Source: CAD feature listing. Evaluate the final solid. Frame: model axes, mm. Face numbers are marked on the shaded views. A direction names the side the tool comes from. Give positions to 0.01 mm unless a question says otherwise; leave off trailing zeros. Order: outer loops, then holes, each group sorted by start corner. A loop starts at its lowest first (then second) coordinate and runs counter-clockwise, first axis right, second up. Notation, with made-up numbers: (74, -17.75) -> (99, -17.75) arc R18 ccw to (99, 7.25) -> close; hole circle Ø1 at (85, 14.5). An arc over 180 degrees is marked (long way). Answer in a Markdown table with one row per item.
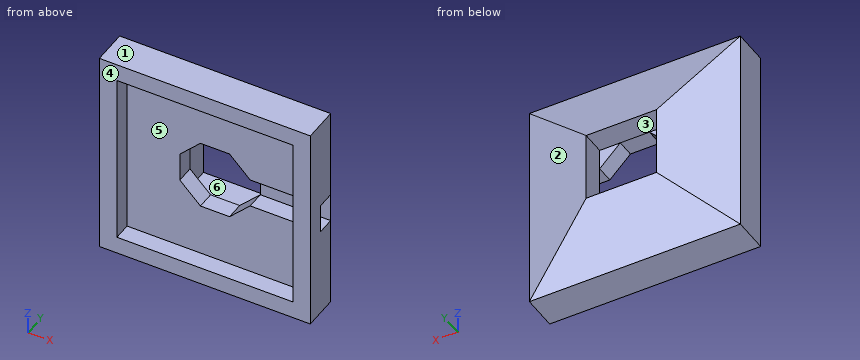
Autodesk Inventor part; units mm, degrees
ref_plane "YZ Plane" through (0, 0, 0) normal (1, 0, 0) x (0, 1, 0)
ref_plane "XZ Plane" through (0, 0, 0) normal (0, 1, 0) x (-1, 0, 0)
ref_plane "XY Plane" through (0, 0, 0) normal (0, 0, 1) x (1, 0, 0)
sketch "Sketch1" plane through (0, 0, 0) normal (0, 1, 0) x (-1, 0, 0)
  line L0 (5, 5) -> (-5, 5)
  line L1 (-5, 5) -> (-5, -5)
  line L2 (-5, -5) -> (5, -5)
  line L3 (5, -5) -> (5, 5)
  line L4 (6, 6) -> (-6, 6)
  line L5 (-6, 6) -> (-6, -6)
  line L6 (-6, -6) -> (6, -6)
  line L7 (6, -6) -> (6, 6)
  point P0 (0, 0)
  dimension "d0" = 10
  dimension "d1" = 10
  dimension "d2" = 5
  dimension "d3" = 5
  dimension "d4" = 12
  dimension "d5" = 12
  dimension "d6" = 1
  dimension "d7" = 1
extrude "Extrusion1" add sketch "Sketch1" along normal blind 2
sketch "Sketch2" plane through (6, 0, 6) normal (1, 0, 0) x (0, 0, -1)
  line L0 (0, 0) -> (0, 2)
  line L1 (12, 0) -> (12, 2)
  line L2 (0, 2) -> (12, 2)
  line L3 (12, 2) -> (12, 1)
  line L4 (12, 1) -> (0, 1)
  line L5 (0, 1) -> (0, 2)
  point P0 (6, 0)
extrude "Extrusion2" add sketch "Sketch2" against normal blind 11.5
sketch "Sketch3" plane through (0, 2, 0) normal (0, 1, 0) x (1, 0, 0)
  line L0 (-2, -2) -> (2, -2)
  line L1 (2, -2) -> (2, 2)
  line L2 (2, 2) -> (-2, 2)
  line L3 (-2, 2) -> (-2, -2)
  circle A0 centre (0, 0) radius 2.8284
  line L4 (0, -2.8284) -> (-2.8284, 0)
  line L5 (-2.8284, 0) -> (0, 2.8284)
  line L6 (2.8284, 0) -> (0, 2.8284)
  line L7 (2.8284, 0) -> (0, -2.8284)
  point P0 (0.8284, -2)
  point P1 (2, -0.8284)
  point P2 (2, 0.8284)
  point P3 (0.8284, 2)
  point P4 (-0.8284, 2)
  point P5 (-2, 0.8284)
  point P6 (-2, -0.8284)
  point P7 (-0.8284, -2)
  dimension "d13" = 4
  dimension "d14" = 4
  dimension "d15" = 2
  dimension "d16" = 2
extrude "Extrusion3" cut sketch "Sketch3" along normal blind 23.25 and the other way blind 11.625 contours L4 L3 L5 L2 L6 L1 L7 L0
sketch "Sketch4" plane through (0, 2, 0) normal (0, 1, 0) x (1, 0, 0)
  line L0 (2, -0.8284) -> (2, 0.8284)
  line L1 (2, -0.8284) -> (2.8765, -0.8284)
  line L2 (2.8765, -0.8284) -> (2.8765, 0.8284)
  line L3 (2.8765, 0.8284) -> (2, 0.8284)
  line L4 (2, 0.8284) -> (2, -0.8284)
  line L5 (2.8765, -0.8284) -> (7.5124, -0.8284)
  line L6 (7.5124, -0.8284) -> (7.5124, 0.8284)
  line L7 (7.5124, 0.8284) -> (2.8765, 0.8284)
  line L8 (2.8765, 0.8284) -> (2.8765, -0.8284)
  point P0 (0, 0)
  point P1 (2.8765, 0.8284)
  point P2 (2, 0.8284)
extrude "Extrusion4" cut sketch "Sketch4" against normal blind 1
sketch "Sketch5" plane through (0, 2, 0) normal (0, 1, 0) x (1, 0, 0)
  line L0 (-6, -6) -> (6, -6)
  line L1 (6, 0.8284) -> (6, 6)
  line L2 (-6, -6) -> (6, -6)
  line L3 (6, -6) -> (6, 6)
  line L4 (6, 6) -> (-6, 6)
  line L5 (-6, 6) -> (-6, -6)
  point P0 (0, 0)
  point P1 (6, -6)
extrude "Extrusion5" add sketch "Sketch5" along normal blind 25
sketch "Sketch6" plane through (6, 0, 6) normal (1, 0, 0) x (0, 0, -1)
  line L0 (5.1716, 1) -> (5.1716, 2)
  line L1 (5.1716, 2) -> (-3.596, 2)
  line L2 (0, 0) -> (0, 27)
  line L3 (4, 2) -> (5.1716, 2)
  line L4 (5.1716, 2) -> (16.1787, 2)
  line L5 (5.1716, 2) -> (6.8284, 2)
  line L6 (6, 2) -> (6, 6)
  line L7 (0, 2) -> (6, 4)
  line L8 (6, 4) -> (12, 2)
  line L9 (12, 0) -> (12, 27)
  line L10 (12, 2) -> (-2.4689, 2)
  line L11 (-2.4689, 2) -> (-2.4689, 28.669)
  line L12 (-2.4689, 28.669) -> (12, 28.669)
  line L13 (12, 28.669) -> (12, 2)
  point P0 (6, 0)
  dimension "d23" = 4
extrude "Extrusion6" cut sketch "Sketch6" against normal blind 23.25 contours L1 L11 L12 L13 L9 L8 L7
sketch "Sketch7" plane through (-6, 0, 6) normal (0, 0, 1) x (1, 0, 0)
  line L0 (6, 0) -> (6, 4)
  line L1 (12, 4) -> (0, 4)
  line L2 (0, 2) -> (12, 2)
  line L3 (12, 2) -> (6, 4)
  line L4 (0, 4) -> (0, 2)
  line L5 (6, 4) -> (0, 2)
  line L6 (0, 2) -> (13.6732, 2)
  line L7 (13.6732, 2) -> (13.6732, 4.9606)
  line L8 (13.6732, 4.9606) -> (0, 4.9606)
  line L9 (0, 4.9606) -> (0, 2)
extrude "Extrusion7" cut sketch "Sketch7" against normal blind 41.75 contours L5 L4 L1 | L1 L9 L8 L7 L6 L3
sketch "Sketch8" plane through (0, 2, 0) normal (0, -1, 0) x (1, 0, 0)
  line L0 (6, 6) -> (0, 0)
  line L1 (1.9974, 1.9974) -> (-2.0026, 1.9974)
  line L2 (-2.0026, 1.9974) -> (-2.0026, -2.0026)
  line L3 (-2.0026, -2.0026) -> (1.9974, -2.0026)
  line L4 (1.9974, -2.0026) -> (1.9974, 1.9974)
  dimension "d30" = 4
  dimension "d31" = 4
extrude "Extrusion8" cut sketch "Sketch8" against normal blind 105
equation "\"BendRadius\" = Thickness"
equation "\"BendReliefWidth\" = Thickness"
equation "\"BendReliefDepth\" = 0.5 * Thickness"
equation "\"CornerReliefSize\" = 4 * Thickness"
equation "\"MinimumRemnant\" = 2 * Thickness"
equation "\"TransitionRadius\" = BendRadius"
equation "\"JacobiRadiusSize\" = BendRadius"
equation "\"GapSize\" = Thickness"
properties part number "modelGatePoklice1"
(1) Access query for the marked faces 4, 5 and 6. Directions: +Z, -Z, +X, -X, +Y, -Y. A direction counts if a zero-diameter tool reaches every point of the face in a straight line with its end or side. Return the directions, or none.
A:
| item | result |
|---|---|
| face 4 | +Z, -Z, +X, -X, -Y |
| face 5 | -Y |
| face 6 | +Y |
(2) Pull-direction query (X, two-part tool) for the marked faces 1, 2 and 3; classes: +X half, -X half, draft (parallel to the pull), parting line (faces both ways), or undercut.
A:
| item | result |
|---|---|
| face 1 | draft |
| face 2 | +X half |
| face 3 | undercut |
(3) First-contact query: pin 1 Ø0.8 at (x, z) = (5.5, -0.5) entering from +Y; pin 2 Ø1.2 at (x, z) = (-0.5, 0) entering from +Y; pin 3 Ø0.8 at (x, z) = (4, 0) entering from -Y. Flat tips, straight axial feed; report the tip coordinate or a pass-through.
A:
| item | result |
|---|---|
| pin 1 | stops at y = 2.3 |
| pin 2 | passes through |
| pin 3 | stops at y = 2 |
(4) Section query B-B (z = 0). Give the number of separate pieces and of enclosed holes in the cut face, plus the area to 3 significant figures.
A:
| item | result |
|---|---|
| separate pieces | 3 |
| enclosed holes | 0 |
| area | 11.3 mm^2 |
(5) Ray query, probe 1 along Z at (x, y) = (0, 1.5); probe 2 along Z at (x, y) = (4, 0.6). Return the intervals inside material, ascending.
A:
| item | result |
|---|---|
| probe 1 | z = -6 to -2, 2 to 6 |
| probe 2 | z = -6 to -5, 5 to 6 |
(6) Section query A-A (y = 2.15). Return the cut outline in (x, z), plus the area to 3 significant figures.
A:
| item | result |
|---|---|
| outline | (-5.55, -5.55) -> (5.55, -5.55) -> (5.55, 5.55) -> (-5.55, 5.55) -> close; hole (-2, -2) -> (2, -2) -> (2, 2) -> (-2, 2) -> close |
| area | 107 mm^2 |
(7) Section query C-C (x = 4.5). Return the cut outline in (y, z).
A:
| item | result |
|---|---|
| outline | (0, -6) -> (2, -6) -> (2.5, -4.5) -> (2.5, 4.5) -> (2, 6) -> (0, 6) -> (0, 5) -> (1, 5) -> (1, 0.83) -> (2, 0.83) -> (2, -0.83) -> (1, -0.83) -> (1, -5) -> (0, -5) -> close |
(8) Section query D-D (z = 1.25). Return the cut outline in (x, y), plus the area to 3 significant figures.
A:
| item | result |
|---|---|
| outline | (-6, 0) -> (-5, 0) -> (-5, 1) -> (-1.58, 1) -> (-1.58, 2) -> (-2, 2) -> (-2, 3.33) -> (-6, 2) -> close; (1.58, 1) -> (5, 1) -> (5, 0) -> (6, 0) -> (6, 2) -> (2, 3.33) -> (2, 2) -> (1.58, 2) -> close |
| area | 16.2 mm^2 |
